Geometry check sheet. Reference: the model listing, model coordinates, mm. Face numbers are marked on the shaded views. A direction names the side the tool comes from. Give positions to 0.01 mm unless a question says otherwise; leave off trailing zeros. Order: outer loops, then holes, each group sorted by start corner. A loop starts at its lowest first (then second) coordinate and runs counter-clockwise, first axis right, second up. Notation, with made-up numbers: M 58.25,-12 L 111.25,-12 A32 ccw 111.25,14 Z; hole C 89,-35.75 d4. An arc over 180 degrees is marked long. Put each result on its own line as item: value. Start each with the question number.
Q1. Go/stop test with flat-tipped pins: pin 1 (2.5 mm diameter, centred on x = -13.5, z = 5.5, fed in from +Y); pin 2 (10 mm diameter, centred on x = -4, z = -5.5, fed in from +Y); pin 3 (1 mm diameter, centred on y = 4, z = -12.5, fed in from -X). Record where each tip stops, or that it passes through.
Q2. Section check A-A on z = 2.5. Record the cut outline in (x, y), then the cut area to 3 significant figures.
Q3. Section check D-D on y = 3. Record the cut outline in (x, z), then the cut area to 3 significant figures.
Q4. Access from +Z, -Z, +X, -X, +Y, -Y to the whole of each face (thin tool, end or side, straight path). Record for the marked faces 3 and 4.
Q5. Material ranges on L1, parallel to Z at x = 2, y = 1.75; L2, parallel to X at y = 1.25, z = -1.5; L3, parallel to Y at x = 3, z = 0, recorded low to high.
Q6. Mould release check, pull along Z, two halves, no side actions. Record for the marked faces 1 and 2: +Z half, -Z half, draft (parallel to the pull), parting line (faces both ways), or undercut.
Q7. Section check B-B on x = -3. Record the cut outline in (y, z).
Q8. Section check C-C on y = 7.25. Record the cut outline in (x, z).
```python
from build123d import *

# Parameters (mm, degrees)
SKETCH1_W             = 68
SKETCH1_H             = 29
BASE_DEPTH            = 2
SKETCH2_R             = 1.5
LEFT_PEG_DEPTH        = 2.5
SKETCH3_R             = 1.5
RIGHT_PEG_DEPTH       = 2.5
SKETCH4_W             = 2
SKETCH4_H             = 14.7
ACCEL_WIRE_HOLE_DEPTH = 2.5
RIGHT_BATTERY_DEPTH   = 1
LEFT_BATTERY_DEPTH    = 1
SKETCH12_R            = 1.25
CUT_EXTRUDE10_DEPTH   = 1.5
SKETCH13_R            = 1.25
CUT_EXTRUDE11_DEPTH   = 1.5
SKETCH14_R            = 2.5
BOSS_EXTRUDE1_DEPTH   = 8


with BuildPart() as part:
    # Sketch1 → base (new body)
    with BuildSketch(Plane(origin=(0, 0, 0), x_dir=(1, 0, 0), z_dir=(0, 1, 0))):
        with Locations((6.444444444, 2.555555556)):
            Rectangle(SKETCH1_W, SKETCH1_H)
    extrude(amount=BASE_DEPTH)

    # Sketch2 → left peg (add)
    with BuildSketch(Plane(origin=(0, 2, 0), x_dir=(1, 0, 0), z_dir=(0, 1, 0))):
        with Locations(Location((-14.155555556, -4.794444444, 0), (0, 0, 270))):
            Circle(SKETCH2_R)
    extrude(amount=LEFT_PEG_DEPTH)

    # Sketch3 → right peg (add)
    with BuildSketch(Plane(origin=(0, 2, 0), x_dir=(1, 0, 0), z_dir=(0, 1, 0))):
        with Locations(Location((-14.155555556, 9.905555556, 0), (0, 0, 270))):
            Circle(SKETCH3_R)
    extrude(amount=RIGHT_PEG_DEPTH)

    # Sketch4 → accel wire hole (cut)
    with BuildSketch(Plane(origin=(0, 2, 0), x_dir=(1, 0, 0), z_dir=(0, 1, 0))):
        with Locations((-24.505555556, 2.555555556)):
            Rectangle(SKETCH4_W, SKETCH4_H)
    extrude(amount=-ACCEL_WIRE_HOLE_DEPTH, mode=Mode.SUBTRACT)

    # Sketch10 → right battery (cut)
    with BuildSketch(Plane(origin=(0, 2, 0), x_dir=(1, 0, 0), z_dir=(0, 1, 0))):
        with BuildLine():
            ThreePointArc((38.444444444, 3.555555556), (20.312137154, 12.950367954), (23.094444444, -7.280841447))
            Line((23.094444444, -7.280841447), (30.794444444, -7.280841447))
            ThreePointArc((30.794444444, -7.280841447), (36.339256843, -3.076751735), (38.444444444, 3.555555556))
        make_face()
        with BuildLine():
            Line((30.794444444, -7.280841447), (23.094444444, -7.280841447))
            ThreePointArc((23.094444444, -7.280841447), (26.944444444, -7.944444444), (30.794444444, -7.280841447))
        make_face()
        with BuildLine():
            ThreePointArc((30.794444444, -7.280841447), (26.944444444, -7.944444444), (23.094444444, -7.280841447))
            Line((23.094444444, -7.280841447), (23.094444444, -10.680841447))
            Line((23.094444444, -10.680841447), (30.794444444, -10.680841447))
            Line((30.794444444, -10.680841447), (30.794444444, -7.280841447))
        make_face()
    extrude(amount=-RIGHT_BATTERY_DEPTH, mode=Mode.SUBTRACT)

    # Sketch11 → left battery (cut)
    with BuildSketch(Plane(origin=(0, 2, 0), x_dir=(1, 0, 0), z_dir=(0, 1, 0))):
        with BuildLine():
            ThreePointArc((5.794444444, 12.391952558), (1.944444444, 13.055555556), (-1.905555556, 12.391952558))
            Line((-1.905555556, 12.391952558), (5.794444444, 12.391952558))
        make_face()
        with BuildLine():
            Line((5.794444444, 12.391952558), (-1.905555556, 12.391952558))
            ThreePointArc((-1.905555556, 12.391952558), (-4.687862846, -7.839256843), (13.444444444, 1.555555556))
            ThreePointArc((13.444444444, 1.555555556), (11.339256843, 8.187862846), (5.794444444, 12.391952558))
        make_face()
        with BuildLine():
            Line((-1.905555556, 15.791952558), (-1.905555556, 12.391952558))
            ThreePointArc((-1.905555556, 12.391952558), (1.944444444, 13.055555556), (5.794444444, 12.391952558))
            Line((5.794444444, 12.391952558), (5.794444444, 15.791952558))
            Line((5.794444444, 15.791952558), (-1.905555556, 15.791952558))
        make_face()
    extrude(amount=-LEFT_BATTERY_DEPTH, mode=Mode.SUBTRACT)

    # Sketch12 → Cut-Extrude10 (cut)
    with BuildSketch(Plane(origin=(0, 1, 0), x_dir=(1, 0, 0), z_dir=(0, 1, 0))):
        with Locations(Location((1.944444444, 14.255555556, 0), (0, 0, 270))):
            Circle(SKETCH12_R)
        with Locations(Location((1.944444444, -6.344444444, 0), (0, 0, 270))):
            Circle(SKETCH12_R)
    extrude(amount=-CUT_EXTRUDE10_DEPTH, mode=Mode.SUBTRACT)

    # Sketch13 → Cut-Extrude11 (cut)
    with BuildSketch(Plane(origin=(0, 1, 0), x_dir=(1, 0, 0), z_dir=(0, 1, 0))):
        with Locations(Location((26.944444444, 11.455555556, 0), (0, 0, 270))):
            Circle(SKETCH13_R)
        with Locations(Location((26.944444444, -9.144444444, 0), (0, 0, 270))):
            Circle(SKETCH13_R)
    extrude(amount=-CUT_EXTRUDE11_DEPTH, mode=Mode.SUBTRACT)

    # Sketch14 → Boss-Extrude1 (add)
    with BuildSketch(Plane(origin=(0, 2, 0), x_dir=(1, 0, 0), z_dir=(0, 1, 0))):
        with Locations(Location((14.444444444, 13.055555556, 0), (0, 0, 270))):
            Circle(SKETCH14_R)
        with Locations(Location((14.444444444, -7.944444444, 0), (0, 0, 270))):
            Circle(SKETCH14_R)
    extrude(amount=BOSS_EXTRUDE1_DEPTH)


solid = part.part
```
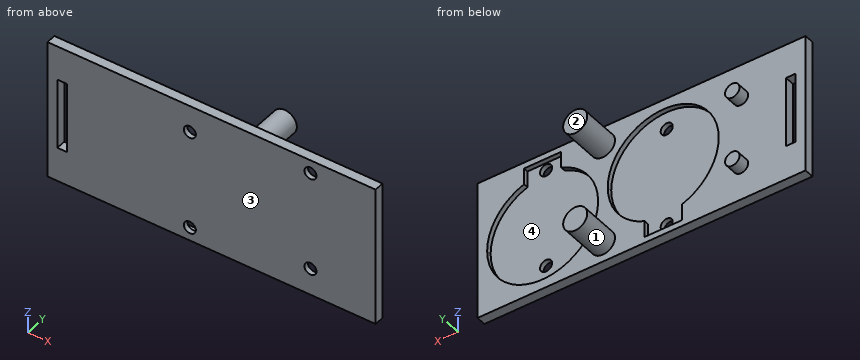
Results found:
1. pin 1: stops at y = 4.5
1. pin 2: stops at y = 2
1. pin 3: stops at x = 11.95
2. outline: M -27.56,0 L -25.51,0 L -25.51,2 L -27.56,2 Z; M -23.51,0 L 40.44,0 L 40.44,2 L 36.72,2 L 36.72,1 L 17.17,1 L 17.17,2 L 12.71,2 L 12.71,1 L -8.82,1 L -8.82,2 L -23.51,2 Z
2. area: 90.9 mm^2
3. outline: C -14.16,-9.91 d3; C -14.16,4.79 d3; C 14.44,-13.06 d5; C 14.44,7.94 d5
3. area: 53.4 mm^2
4. face 3: +Z, -Z, +X, -X, -Y
4. face 4: +Y
5. L1: z = -17.06 to -15.79, 9.94 to 11.94
5. L2: x = -27.56 to -25.51, -23.51 to -9.56, 13.44 to 15.63, 38.26 to 40.44
5. L3: y = 0 to 1
6. face 1: undercut
6. face 2: draft
7. outline: M 0,-17.06 L 2,-17.06 L 2,-11.94 L 1,-11.94 L 1,8.83 L 2,8.83 L 2,11.94 L 0,11.94 Z
8. outline: C 14.44,-13.06 d5; C 14.44,7.94 d5
